Autodesk Inventor part; units mm, degrees
ref_plane "YZ Plane" through (0, 0, 0) normal (1, 0, 0) x (0, 1, 0)
ref_plane "XZ Plane" through (0, 0, 0) normal (0, 1, 0) x (-1, 0, 0)
ref_plane "XY Plane" through (0, 0, 0) normal (0, 0, 1) x (1, 0, 0)
sketch "Sketch1" plane through (0, 0, 0) normal (0, 1, 0) x (-1, 0, 0)
  line L0 (15.9, 17.35) -> (-15.9, 17.35)
  line L1 (-15.9, 17.35) -> (-15.9, -17.35)
  line L2 (-15.9, -17.35) -> (15.9, -17.35)
  line L3 (15.9, -17.35) -> (15.9, 17.35)
  line L4 (15.9, 17.35) -> (-15.9, -17.35) construction
  line L5 (-15.9, 17.35) -> (15.9, -17.35) construction
  circle A0 centre (13.775, 14.825) radius 1.375
  line L6 (0, 17.35) -> (0, -17.35) construction
  line L7 (15.9, 0) -> (-15.9, 0) construction
  circle A1 centre (13.775, -14.825) radius 1.375
  circle A2 centre (-13.775, 14.825) radius 1.375
  circle A3 centre (-13.775, -14.825) radius 1.375
  point P0 (0, 0)
  dimension "d0" = 31.8
  dimension "d1" = 34.7
  dimension "d2" = 2.75
  dimension "d3" = 2.125
  dimension "d4" = 2.525
extrude "Extrusion1" add sketch "Sketch1" along normal blind 1
properties part number "motordriver_footprint"
The model under review builds one solid part; all positions refer to its coordinate system, in mm. Round coordinates to 2 decimals unless told otherwise and drop trailing zeros. Loops run counter-clockwise (first coordinate to the right, second up) from the corner with the lowest first, then second, coordinate; pieces in that order, holes last. Notation, with made-up numbers: (-15, 71) -> (-2, 71) arc R23 cw to (-2, 80) -> close; hole circle Ø2 at (-19.5, 34). An arc over 180 degrees is marked (long way). Write item = value, one per line. Start each with the question number.
Item 1: To check wall thickness, follow L1, parallel to Z at x = 13, y = 0.15; L2, parallel to X at y = 0.5, z = 14 (3 decimals); L3, parallel to Z at x = 13.5, y = 0.1. State the ranges of each line that lie inside material, in increasing order.
Item 2: Mouldability with a two-part tool opening along Z and no side actions: class faces 1 (the cylindrical face through (-15.045, 0.493, -14.298)), 2 (the flat face through (0.2, 0.5, -17.35)), 3 (the flat face through (15.9, 0.5, 0.2)) as released by +Z, released by -Z, zero draft, split by the parting line, or undercut.
Item 3: Take a section at A-A on y = 0.15. Give the boundary of the cut face in (x, z) (3 decimals).
Item 4: Insertion check: pin 1 (2.5 mm diameter, centred on x = -13.775, z = 14.825, fed in from -Y). The pin has a flat end and moves straight along its axis. Give the tip position at first contact, or say it passes through.
Result:
q1.L1 = -17.35 to -15.96, -13.69 to 13.69, 15.96 to 17.35
q1.L2 = -15.9 to -14.875, -12.675 to 12.675, 14.875 to 15.9
q1.L3 = -17.35 to -16.17, -13.48 to 13.48, 16.17 to 17.35
q2.face_1 = undercut
q2.face_2 = released by -Z
q2.face_3 = zero draft
q3.outline = (-15.9, -17.35) -> (15.9, -17.35) -> (15.9, 17.35) -> (-15.9, 17.35) -> close; hole circle Ø2.75 at (-13.775, -14.825); hole circle Ø2.75 at (-13.775, 14.825); hole circle Ø2.75 at (13.775, -14.825); hole circle Ø2.75 at (13.775, 14.825)
q4.pin_1 = through
